Answer from the drawing. Dimensions are ordinates in mm from the lowest x, y and z of the part. A direction names the side the tool comes from. Coordinates: 2 decimals unless noted, no trailing zeros. Order: outer loops, then holes, each group sorted by start corner. A loop starts at its lowest first (then second) coordinate and runs counter-clockwise, first axis right, second up. Notation, with made-up numbers: (-15.75, 37) -> (6.25, 37) arc R28 cw to (6.25, 59) -> close; hole circle Ø2 at (34, 36). An arc over 180 degrees is marked (long way). Answer in a Markdown table with one row per item.
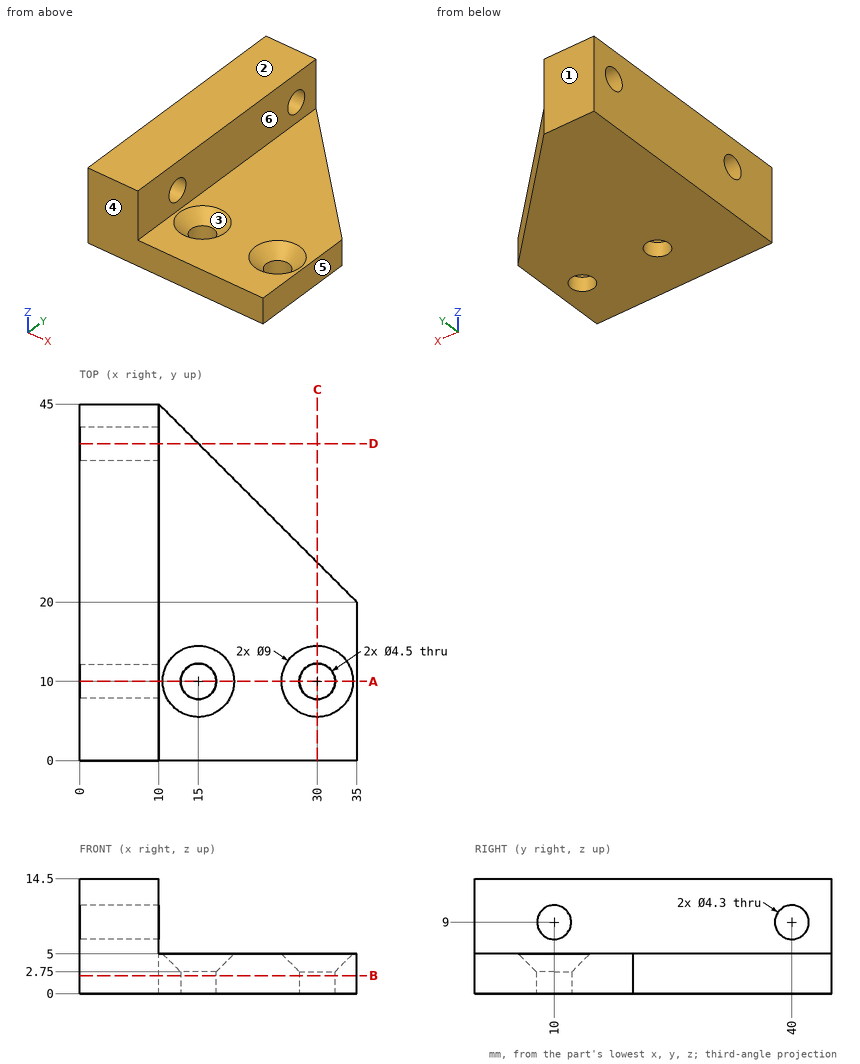
Q1. The part is cut by section C-C (x = 30). Write down the section's boundary in (y, z).
Outcome:
| item | result |
|---|---|
| outline | (0, 0) -> (7.75, 0) -> (7.75, 2.75) -> (5.5, 5) -> (0, 5) -> close; (12.25, 0) -> (25, 0) -> (25, 5) -> (14.5, 5) -> (12.25, 2.75) -> close |
Q2. Given pin 1 (12.5 mm diameter, centred on x = 27, y = 17.5, fed in from +Z), flat-ended and moving along its own axis, determine where the tip first touches the part or whether it passes through.
Outcome:
| item | result |
|---|---|
| pin 1 | z = 5 |
Q3. The part is cut by section D-D (y = 40). Write down the section's boundary in (x, z), then the cut area to 3 significant figures.
Outcome:
| item | result |
|---|---|
| outline | (0, 0) -> (15, 0) -> (15, 5) -> (10, 5) -> (10, 6.85) -> (0, 6.85) -> close; (0, 11.15) -> (10, 11.15) -> (10, 14.5) -> (0, 14.5) -> close |
| area | 127 mm² |
Q4. The part is cut by section B-B (z = 2.25). Write down the section's boundary in (x, y).
Outcome:
| item | result |
|---|---|
| outline | (0, 0) -> (35, 0) -> (35, 20) -> (10, 45) -> (0, 45) -> close; hole circle Ø4.5 at (15, 10); hole circle Ø4.5 at (30, 10) |
Q5. For the marked faces 5 and 6, determine the directions among +Z, -Z, +X, -X, +Y, -Y from which every point of the face is accessible in a straight line to the end or side of a thin tool.
Outcome:
| item | result |
|---|---|
| face 5 | +Z, -Z, +X, +Y, -Y |
| face 6 | +Z, +X, +Y, -Y |
Q6. Consider line 1 (X direction, y = 10, z = 2.1); line 2 (Z direction, x = 3, y = 10); line 3 (Y direction, x = 2, z = 8.5). Determine where each line is inside the solid, lowest interval first.
Outcome:
| item | result |
|---|---|
| line 1 | 0 to 12.75, 17.25 to 27.75, 32.25 to 35 |
| line 2 | 0 to 6.85, 11.15 to 14.5 |
| line 3 | 0 to 7.91, 12.09 to 37.91, 42.09 to 45 |
Q7. The part is cut by section A-A (y = 10). Write down the section's boundary in (x, z), then the cut area to 3 significant figures.
Outcome:
| item | result |
|---|---|
| outline | (0, 0) -> (12.75, 0) -> (12.75, 2.75) -> (10.5, 5) -> (10, 5) -> (10, 6.85) -> (0, 6.85) -> close; (0, 11.15) -> (10, 11.15) -> (10, 14.5) -> (0, 14.5) -> close; (17.25, 0) -> (27.75, 0) -> (27.75, 2.75) -> (25.5, 5) -> (19.5, 5) -> (17.25, 2.75) -> close; (32.25, 0) -> (35, 0) -> (35, 5) -> (34.5, 5) -> (32.25, 2.75) -> close |
| area | 172 mm² |
Q8. For a pull along Y with two mould halves and no side action, classify the marked faces 1, 2, 3 and 4 as pulls with the +Y half, pulls with the -Y half, needs draft (parallel to the pull), parting line crosses it, or undercut.
Outcome:
| item | result |
|---|---|
| face 1 | pulls with the +Y half |
| face 2 | needs draft |
| face 3 | undercut |
| face 4 | pulls with the -Y half |
